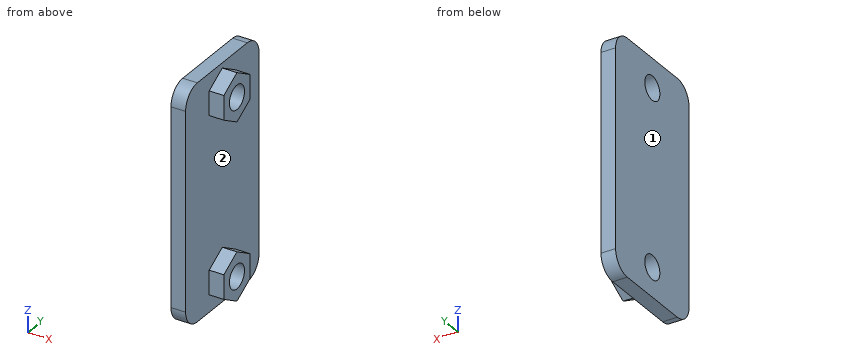
```python
from build123d import *

# Parameters (mm, degrees)
SZKIC2_W                    = 80
SZKIC2_H                    = 40
DODANIE_WYCI_GNI_CIE1_DEPTH = 5
ZAOKR_GLENIE1_R             = 6.4
SZKIC3_R                    = 4.1
WYTNIJ_WYCI_GNI_CIE1_DEPTH  = 10
DODANIE_WYCI_GNI_CIE2_DEPTH = 5
WYTNIJ_WYCI_GNI_CIE2_START  = -15
SZKIC5_R                    = 4.1
WYTNIJ_WYCI_GNI_CIE2_DEPTH  = 15


with BuildPart() as part:
    # Szkic2 → Dodanie-wyciągnięcie1 (new body)
    with BuildSketch(Plane(origin=(0, 0, 0), x_dir=(0, 0, -1), z_dir=(1, 0, 0))):
        Rectangle(SZKIC2_W, SZKIC2_H)
    extrude(amount=DODANIE_WYCI_GNI_CIE1_DEPTH)

    # Zaokrąglenie1
    zaokr_glenie1_edges = [part.edges().sort_by_distance(p)[0] for p in [
        (2.5, -20, -40),
        (2.5, -20, 40),
        (2.5, 20, 40),
        (2.5, 20, -40),
    ]]
    fillet(zaokr_glenie1_edges, radius=ZAOKR_GLENIE1_R)

    # Szkic3 → Wytnij-wyciągnięcie1 (cut, symmetric)
    with BuildSketch(Plane(origin=(5, 0, 0), x_dir=(0, 0, -1), z_dir=(1, 0, 0))):
        with Locations((-30, 0)):
            Circle(SZKIC3_R)
        with Locations((30, 0)):
            Circle(SZKIC3_R)
    extrude(amount=WYTNIJ_WYCI_GNI_CIE1_DEPTH, both=True, mode=Mode.SUBTRACT)

    # Szkic4 → Dodanie-wyciągnięcie2 (add)
    with BuildSketch(Plane(origin=(5, 0, 0), x_dir=(0, 0, -1), z_dir=(1, 0, 0))):
        Polygon((-21.743891151, 0), (-25.871945575, 7.15), (-34.128054425, 7.15), (-38.256108849, 0), (-34.128054425, -7.15), (-25.871945575, -7.15), align=None)
        Polygon((21.743891151, 0), (25.871945575, -7.15), (34.128054425, -7.15), (38.256108849, 0), (34.128054425, 7.15), (25.871945575, 7.15), align=None)
    extrude(amount=DODANIE_WYCI_GNI_CIE2_DEPTH)

    # Szkic5 → Wytnij-wyciągnięcie2 (cut)
    with BuildSketch(Plane.ZY.offset(WYTNIJ_WYCI_GNI_CIE2_START)):
        with Locations(Location((30, 0, 0), (0, 0, 180))):
            Circle(SZKIC5_R)
        with Locations(Location((-30, 0, 0), (0, 0, 180))):
            Circle(SZKIC5_R)
    extrude(amount=WYTNIJ_WYCI_GNI_CIE2_DEPTH, mode=Mode.SUBTRACT)


solid = part.part
```
Part model, mm, in its own coordinate system. Face numbers are marked on the shaded views. Give positions to 0.01 mm unless a question says otherwise; leave off trailing zeros. Order: outer loops, then holes, each group sorted by start corner. A loop starts at its lowest first (then second) coordinate and runs counter-clockwise, first axis right, second up. Notation, with made-up numbers: (9, 37.25) - (25, 37.25) arc R28 ccw to (25, 68.25) - close; hole circle Ø6 at (33, -3.75). An arc over 180 degrees is marked (long way). Use one line per item in the form item = value.
Item 1: Two-plate mould, pull along Z, no slides. Class the marked faces 1 and 2: released by +Z, released by -Z, zero draft, split by the parting line, or undercut.
Solution:
face_1 = zero draft
face_2 = undercut
Item 2: Slice it at C-C on y = -2. Give the cut face in (x, z), and give its area (3 significant figures).
Solution:
outline = (0, -40) - (5, -40) - (5, -37.1) - (10, -37.1) - (10, -33.58) - (0, -33.58) - close; (0, -26.42) - (10, -26.42) - (10, -22.9) - (5, -22.9) - (5, 22.9) - (10, 22.9) - (10, 26.42) - (0, 26.42) - close; (0, 33.58) - (10, 33.58) - (10, 37.1) - (5, 37.1) - (5, 40) - (0, 40) - close
area = 399 mm2
Item 3: Probe probe 1 along Y at (x, z) = (2.5, 30); probe 2 along Y at (x, z) = (7, 30); probe 3 along Z at (x, y) = (3, -0.5). List the from-to ranges inside material, lowest first. Write a range as from..to.
Solution:
probe_1 = -20..-4.1, 4.1..20
probe_2 = -7.15..-4.1, 4.1..7.15
probe_3 = -40..-34.07, -25.93..25.93, 34.07..40
Item 4: Pin check, flat tips, straight feed: pin 1 Ø2 at (y, z) = (-10.5, 20.5) entering from -X; pin 2 Ø12 at (y, z) = (-5, 14.5) entering from +X; pin 3 Ø1.5 at (x, z) = (7, 29.5) entering from -Y; pin 4 Ø2.5 at (x, z) = (6.5, -30.5) entering from +Y. Stop position of each tip, or through.
Solution:
pin_1 = 0
pin_2 = 5
pin_3 = -7.15
pin_4 = 7.15
Item 5: Slice it at A-A on x = 6.5. Give the cut face in (y, z).
Solution:
outline = (-7.15, -34.13) - (0, -38.26) - (7.15, -34.13) - (7.15, -25.87) - (0, -21.74) - (-7.15, -25.87) - close; (-7.15, 25.87) - (0, 21.74) - (7.15, 25.87) - (7.15, 34.13) - (0, 38.26) - (-7.15, 34.13) - close; hole circle Ø8.2 at (0, -30); hole circle Ø8.2 at (0, 30)
Item 6: Slice it at D-D on y = 9. Give the cut face in (x, z), and give its area (3 significant figures).
Solution:
outline = (0, -40) - (5, -40) - (5, 40) - (0, 40) - close
area = 400 mm2
Item 7: Slice it at B-B on z = 30. Give the cut face in (x, y), and give its area (4 significant figures).
Solution:
outline = (0, -20) - (5, -20) - (5, -7.15) - (10, -7.15) - (10, -4.1) - (0, -4.1) - close; (0, 4.1) - (10, 4.1) - (10, 7.15) - (5, 7.15) - (5, 20) - (0, 20) - close
area = 189.5 mm2
